```python
from build123d import *

# Parameters (mm, degrees)
F1_DEPTH = 7
F2_W     = 11
F2_H     = 13.5
F3_DEPTH = 8
F4_W     = 22
F4_H     = 12
F5_DEPTH = 11.5
F6_W     = 3
F6_H     = 2
F7_DEPTH = 1
F6_W_2   = 6.2
F6_H_2   = 6.3
F6_W_3   = 6
F6_H_3   = 3.6
F8_DEPTH = 5


with BuildPart() as f1:
    # F0 (on Top) → F1 (new body)
    with BuildSketch(Plane.XY):
        Polygon((4.890249, 40.097855), (-36.109751, 40.097855), (-36.109751, 22.697855), (-33.109751, 22.697855), (-33.109751, 1.697855), (-36.109751, 1.697855), (-36.109751, -15.902145), (4.890249, -15.902145), (4.890249, 1.697855), (1.890249, 1.697855), (1.890249, 22.697855), (4.890249, 22.697855), align=None)
    extrude(amount=F1_DEPTH)

    # F2 (on face) → F3 (join)
    with BuildSketch(Plane.XY.offset(7)):
        with Locations((-0.609751, -9.152145)):
            Rectangle(F2_W, F2_H)
    extrude(amount=F3_DEPTH)

    # F4 (on face) → F5 (join)
    with BuildSketch(Plane.XY.offset(7)):
        with Locations((-20.609751, -2.402145)):
            Rectangle(F4_W, F4_H)
    extrude(amount=F5_DEPTH)

    # F6 (on face) → F7 (join)
    with BuildSketch(Plane.XY.offset(18.5)):
        with Locations((-13.109751, 0.397855)):
            Rectangle(F6_W, F6_H)
    extrude(amount=F7_DEPTH)

    # F6 (on face) → F8 (join)
    with BuildSketch(Plane.XY.offset(18.5)):
        with Locations((-25.909751, -2.452145)):
            Rectangle(F6_W_2, F6_H_2)
        with Locations((-16.609751, -6.402145)):
            Rectangle(F6_W_3, F6_H_3)
    extrude(amount=F8_DEPTH)


solid = f1.part
```
Geometry check sheet. Reference: the model listing, model coordinates, mm. A direction names the side the tool comes from. Round coordinates to 2 decimals unless told otherwise and drop trailing zeros. Write each loop counter-clockwise with the first axis right and the second up, starting at its lowest first coordinate (ties: lowest second). Pieces come first, ordered by that corner, then holes. Notation, with made-up numbers: (38, 24.25) -> (64, 24.25) arc R21 ccw to (64, 54.25) -> close; hole circle Ø1 at (59, 83). An arc over 180 degrees is marked (long way). Put each result on its own line as item: value.
1) Cross-section at B-B, the plane x = -17. Enter the section's corners in (y, z).
Recorded:
outline: (-15.9, 0) -> (40.1, 0) -> (40.1, 7) -> (3.6, 7) -> (3.6, 18.5) -> (-4.6, 18.5) -> (-4.6, 23.5) -> (-8.2, 23.5) -> (-8.2, 18.5) -> (-8.4, 18.5) -> (-8.4, 7) -> (-15.9, 7) -> close
2) Cross-section at D-D, the plane z = 2.75. Enter the section's corners in (x, y), plus the area to 3 significant figures.
Recorded:
outline: (-36.11, -15.9) -> (4.89, -15.9) -> (4.89, 1.7) -> (1.89, 1.7) -> (1.89, 22.7) -> (4.89, 22.7) -> (4.89, 40.1) -> (-36.11, 40.1) -> (-36.11, 22.7) -> (-33.11, 22.7) -> (-33.11, 1.7) -> (-36.11, 1.7) -> close
area: 2,170 mm2
3) Access from +Z, -Z, +X, -X, +Y, -Y to the whole of each face (thin tool, end or side, straight path). Record for faces 1 (the face through (-1, -2.402, 11)), 2 (the face through (-6.11, -9, 11)), 3 (the face through (-21, 3.598, 13)).
Recorded:
face 1: +Z, +X, +Y
face 2: +Z, +Y, -Y
face 3: +Z, +X, -X, +Y
4) Thickness scan on probe 1 along X at (y, z) = (-7.5, 8); probe 2 along Z at (x, y) = (-27.5, -6); probe 3 along Z at (x, y) = (-15, 15). Record the ranges inside material, lowest first. Write a range as from..to.
Recorded:
probe 1: x = -31.61..-9.61, -6.11..4.89
probe 2: z = 0..18.5
probe 3: z = 0..7
5) Release check for a two-part mould opening along Y. For faces 4 (the face through (-26, -5.602, 21)), 5 (the face through (-35, 1.698, 3)), 6 (the face through (-29.01, -2, 21)) record: pulls with the +Y half, pulls with the -Y half, needs draft (parallel to the pull), parting line crosses it, or undercut.
Recorded:
face 4: pulls with the -Y half
face 5: undercut
face 6: needs draft
6) Cross-section at C-C, the plane y = -6.5. Enter the section's corners in (x, z).
Recorded:
outline: (-36.11, 0) -> (4.89, 0) -> (4.89, 15) -> (-6.11, 15) -> (-6.11, 7) -> (-9.61, 7) -> (-9.61, 18.5) -> (-13.61, 18.5) -> (-13.61, 23.5) -> (-19.61, 23.5) -> (-19.61, 18.5) -> (-31.61, 18.5) -> (-31.61, 7) -> (-36.11, 7) -> close
7) Depth check by flat-ended pin: P1, Ø1.5, axis at y = -3.5, z = 20, coming from the -X side; P2, Ø2.5, axis at y = -11.5, z = 12.5, coming from the -X side; P3, Ø5.5, axis at x = -24.5, z = 21.5, coming from the +Y side. Enter the tip coordinate at first touch or a pass-through.
Recorded:
P1: stops at x = -29.01
P2: stops at x = -6.11
P3: stops at y = 0.7
8) Cross-section at A-A, the plane z = 20.5. Enter the section's corners in (x, y), plus the area to 3 significant figures.
Recorded:
outline: (-29.01, -5.6) -> (-22.81, -5.6) -> (-22.81, 0.7) -> (-29.01, 0.7) -> close; (-19.61, -8.2) -> (-13.61, -8.2) -> (-13.61, -4.6) -> (-19.61, -4.6) -> close
area: 60.7 mm2
